Design review of the part built by this model. Coordinates are the model's own, in mm. Give positions to 0.01 mm unless a question says otherwise; leave off trailing zeros. Write each loop counter-clockwise with the first axis right and the second up, starting at its lowest first coordinate (ties: lowest second). Pieces come first, ordered by that corner, then holes. Notation, with made-up numbers: M 81.5,50 L 88.5,50 A22 ccw 88.5,76 Z; hole C 22,33.25 d11. An arc over 180 degrees is marked long. Write each question's results on one line, items separated by ' | '. Start each with the question number.
from build123d import *

# Parameters (mm, degrees)
SKETCH1_W               = 40
SKETCH1_H               = 71.5
SKETCH1_R               = 6.5
BOSS_EXTRUDE1_DEPTH     = 3.175
CHAMFER1_SIZE           = 4
SKETCH2_R               = 1.875
CUT_EXTRUDE1_DEPTH      = 4.175
F_1_4_CLEARANCE_HOLE1_D = 6.5278


with BuildPart() as part:
    # Sketch1 → Boss-Extrude1 (new body)
    with BuildSketch(Plane.XY):
        with Locations((0, -6.75)):
            Rectangle(SKETCH1_W, SKETCH1_H)
        Circle(SKETCH1_R, mode=Mode.SUBTRACT)
    extrude(amount=BOSS_EXTRUDE1_DEPTH)

    # Chamfer1
    chamfer1_edges = [part.edges().sort_by_distance(p)[0] for p in [
        (-20, 29, 1.5875),
        (20, 29, 1.5875),
        (20, -42.5, 1.5875),
        (-20, -42.5, 1.5875),
    ]]
    chamfer(chamfer1_edges, length=CHAMFER1_SIZE)

    # Sketch2 → Cut-Extrude1 (cut, through all)
    with BuildSketch(Plane.XY.offset(3.175)):
        with Locations((-7.75, 6.524250301)):
            Circle(SKETCH2_R)
        with Locations((7.75, 6.524250301)):
            Circle(SKETCH2_R)
        with Locations((15.5, -6.899143458)):
            Circle(SKETCH2_R)
        with Locations((7.75, -20.322537216)):
            Circle(SKETCH2_R)
        with Locations((-7.75, -20.322537216)):
            Circle(SKETCH2_R)
        with Locations((-15.5, -6.899143458)):
            Circle(SKETCH2_R)
    extrude(amount=-CUT_EXTRUDE1_DEPTH, mode=Mode.SUBTRACT)

    # 1/4 Clearance Hole1 (through all)
    with Locations(Plane(origin=(0, 0, 0), x_dir=(-1, 0, 0), z_dir=(0, 0, -1))):
        with Locations((-11.684, 21.299580024), (2.54, 21.299580024), (-11.684, -34.580419976), (2.54, -34.580419976)):
            Hole(F_1_4_CLEARANCE_HOLE1_D / 2)


solid = part.part
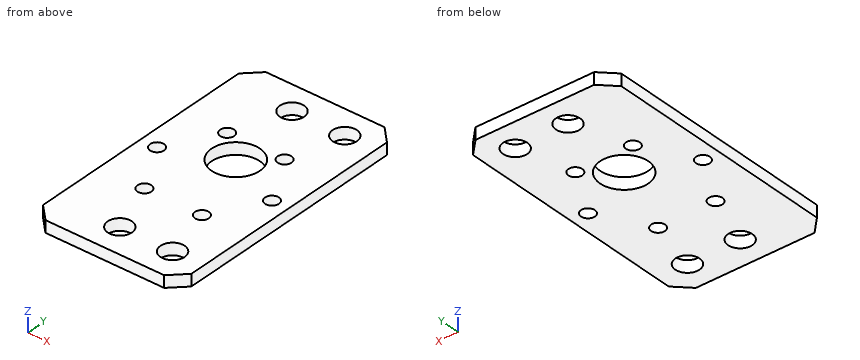
Q1. For pin 1 Ø3 at (x, y) = (7.75, -20.32) entering from +Z, flat-tipped, find the tip position at first contact; note if it passes through.
Q2. We need section D-D on x = -2.54. Write out the cut boundary in (y, z) (3 decimals).
Q3. We need section C-C on z = 0.7. Count the separate pieces of the cut face and the enclosed holes in it, and give its area (3 significant figures).
Q4. We need section A-A on x = 7.75. Write out the cut boundary in (y, z) (3 decimals), and give its area (3 significant figures).
Q5. Wall thickness on line 1 along Y through (x, z) = (8, 3); line 2 along Y through (x, z) = (-7.75, 1.8); line 3 along X through (y, z) = (-33.5, 0.65): over which ranges is each line inside the solid? List them lowest first. Write a range as from..to.
Q6. We need section B-B on y = 0. Write out the cut boundary in (x, z) (3 decimals), and give its area (3 significant figures).
Answer sheet:
1) pin 1: through
2) outline: M -42.5,0 L -37.844,0 L -37.844,3.175 L -42.5,3.175 Z; M -31.317,0 L -5.983,0 L -5.983,3.175 L -31.317,3.175 Z; M 5.983,0 L 18.036,0 L 18.036,3.175 L 5.983,3.175 Z; M 24.563,0 L 29,0 L 29,3.175 L 24.563,3.175 Z
3) separate pieces: 1 | enclosed holes: 11 | area: 2,500 mm^2
4) outline: M -42.5,0 L -22.198,0 L -22.198,3.175 L -42.5,3.175 Z; M -18.448,0 L 4.649,0 L 4.649,3.175 L -18.448,3.175 Z; M 8.399,0 L 29,0 L 29,3.175 L 8.399,3.175 Z | area: 203 mm^2
5) line 1: -42.5..-22.18, -18.46..4.67, 8.38..29 | line 2: -42.5..-22.2, -18.45..4.65, 8.4..29 | line 3: -20..-5.62, 0.54..8.6, 14.76..20
6) outline: M -20,0 L -6.5,0 L -6.5,3.175 L -20,3.175 Z; M 6.5,0 L 20,0 L 20,3.175 L 6.5,3.175 Z | area: 85.7 mm^2
